```python
from build123d import *

# Parameters (mm, degrees)
CHAMFER_1_SIZE = 0.5


with BuildPart() as part:
    # Sketch 1 → Revolve 1 (revolve)
    with BuildSketch(Plane.XY, mode=Mode.PRIVATE) as revolve_1_sk:
        Polygon((-40, 20), (-40, 0), (-15, 0), (-15, 6), (-38.5, 6), (-38.5, 8), (-37, 8), (-37, 20), align=None)
    revolve(revolve_1_sk.sketch.rotate(Axis((0, 26.168985987, 0), (0, -1, 0)), 270), axis=Axis((0, 26.168985987, 0), (0, -1, 0)))

    # Chamfer 1
    chamfer_1_edges = [part.edges().sort_by_distance(p)[0] for p in [
        (0, 20, -40),
        (0, 20, -37),
        (0, 0, -15),
        (0, 0, -40),
    ]]
    chamfer(chamfer_1_edges, length=CHAMFER_1_SIZE)


solid = part.part
```
Can you work these out from the model? Positions are in its coordinate system, mm. A direction names the side the tool comes from. Coordinates: 2 decimals unless noted, no trailing zeros. Loops run counter-clockwise (first coordinate to the right, second up) from the corner with the lowest first, then second, coordinate; pieces in that order, holes last.
Item 1: Suppose I cut it at D-D (y = 18). Please give me the cut outline in (x, z), then the cut area to 3 significant figures.
Answers below:
outline: circle Ø80 at (0, 0); hole circle Ø74 at (0, 0)
area: 726 mm2
Item 2: Suppose I cut it at B-B (z = 0). Please give me the cut outline in (x, y), then the cut area to 3 significant figures.
Answers below:
outline: (-40, 0.5) - (-39.5, 0) - (-15.5, 0) - (-15, 0.5) - (-15, 6) - (-38.5, 6) - (-38.5, 8) - (-37, 8) - (-37, 19.5) - (-37.5, 20) - (-39.5, 20) - (-40, 19.5) - close; (15, 0.5) - (15.5, 0) - (39.5, 0) - (40, 0.5) - (40, 19.5) - (39.5, 20) - (37.5, 20) - (37, 19.5) - (37, 8) - (38.5, 8) - (38.5, 6) - (15, 6) - close
area: 377 mm2
Item 3: If we mould it in two halves opening along X, with no side actions, what happens to faces 4 (the face through (39.05, 9.87, -8.67)), 5 (the face through (37.584, 7.014, -8.346)), 6 (the face through (14, 20, -35))? For each: released by +X, released by -X, zero draft, split by the parting line, or undercut.
Answers below:
face 4: split by the parting line
face 5: undercut
face 6: zero draft
Item 4: Suppose I cut it at A-A (x = 0). Please give me the cut outline in (y, z), then the cut area to 3 significant figures.
Answers below:
outline: (0, -39.5) - (0.5, -40) - (19.5, -40) - (20, -39.5) - (20, -37.5) - (19.5, -37) - (8, -37) - (8, -38.5) - (6, -38.5) - (6, -15) - (0.5, -15) - (0, -15.5) - close; (0, 15.5) - (0.5, 15) - (6, 15) - (6, 38.5) - (8, 38.5) - (8, 37) - (19.5, 37) - (20, 37.5) - (20, 39.5) - (19.5, 40) - (0.5, 40) - (0, 39.5) - close
area: 377 mm2
Item 5: Please list where these lines run through material, in increasing order: L1, parallel to X at y = 3.9, z = 0; L2, parallel to X at y = 11.5, z = 0; L3, parallel to Y at x = 9, z = 17.
Answers below:
L1: x = -40 to -15, 15 to 40
L2: x = -40 to -37, 37 to 40
L3: y = 0 to 6
Item 6: I'm going to push flat-ended pins straight in: pin 1 (10 mm diameter, centred on x = 25, z = 17.5, fed in from +Y); pin 2 (12 mm diameter, centred on x = -11, y = 10, fed in from +Z); pin 3 (5 mm diameter, centred on x = -14.5, y = 4.5, fed in from +Z); pin 4 (18 mm diameter, centred on x = 0, z = 0, fed in from +Y). Where does each tip first touch, or does it pass through?
Answers below:
pin 1: stops at y = 6
pin 2: stops at z = 39.69
pin 3: stops at z = 38.16
pin 4: passes through
Item 7: Which directions (+Z, -Z, +X, -X, +Y, -Y) give clear straight access to the entire face, cutting with the end or side of a thin tool? Please do faces 1 (the face through (-32, 8, -20)), 2 (the face through (-1, 0, 17)), 3 (the face through (14.17, 13.83, 34.18)).
Answers below:
face 1: none
face 2: +Z, -Z, +X, -X, -Y
face 3: +Y
Item 8: Suppose I cut it at C-C (y = 2). Please give me the cut outline in (x, z).
Answers below:
outline: circle Ø80 at (0, 0); hole circle Ø30 at (0, 0)
